```python
from build123d import *

# Parameters (mm, degrees)
BOSS_EXTRUDE1_DEPTH = 12
CUT_EXTRUDE1_DEPTH  = 20


with BuildPart() as part:
    # Sketch1 → Boss-Extrude1 (new body)
    with BuildSketch(Plane(origin=(0, 0, 0), x_dir=(1, 0, 0), z_dir=(0, 1, 0))):
        Polygon((0, 7.38), (-6.39126748, 3.69), (-6.39126748, -3.69), (0, -7.38), (6.39126748, -3.69), (6.39126748, 3.69), align=None)
    extrude(amount=BOSS_EXTRUDE1_DEPTH)

    # Sketch2 → Cut-Extrude1 (cut)
    with BuildSketch(Plane.XZ):
        Polygon((-2.165063509, -1.25), (2.165063509, -1.25), (0, 2.5), align=None)
    extrude(amount=-CUT_EXTRUDE1_DEPTH, mode=Mode.SUBTRACT)


solid = part.part
```
Verification items for the finished model (mm, model axes). A direction names the side the tool comes from. Coordinates: 2 decimals unless noted, no trailing zeros. Order: outer loops, then holes, each group sorted by start corner. A loop starts at its lowest first (then second) coordinate and runs counter-clockwise, first axis right, second up. Notation, with made-up numbers: (63, 12.5) - (79, 12.5) arc R21 cw to (79, 51.5) - close; hole circle Ø10 at (55, -30). An arc over 180 degrees is marked (long way). Return JSON: item names as keys, results as strings.
(1) Go/stop test with flat-tipped pins: pin 1 (6 mm diameter, centred on x = -1, y = 3, fed in from +Z); pin 2 (6 mm diameter, centred on x = -3.5, y = 9.5, fed in from -Z); pin 3 (5 mm diameter, centred on x = 3.5, z = -5.5, fed in from -Y). Record where each tip stops, or that it passes through.
Filled sheet:
{"pin 1": "stops at z = 7.38", "pin 2": "stops at z = -7.09", "pin 3": "stops at y = 0"}
(2) Mould release check, pull along X, two halves, no side actions. Record for faces 1 (the flat face through (-2, 0, 0)), 2 (the flat face through (3.24, 5.92, -5.51)), 3 (the flat face through (-1.07, 5.92, 0.65)): pulls with the +X half, pulls with the -X half, needs draft (parallel to the pull), parting line crosses it, or undercut.
Filled sheet:
{"face 1": "needs draft", "face 2": "pulls with the +X half", "face 3": "undercut"}
(3) Thickness scan on line 1 along Z through (x, y) = (-1, 1); line 2 along Z through (x, y) = (0.25, 4.5); line 3 along X through (y, z) = (2, 1.5). Record the ranges inside material, lowest first.
Filled sheet:
{"line 1": "z = -6.8 to -1.25, 0.77 to 6.8", "line 2": "z = -7.24 to -1.25, 2.07 to 7.24", "line 3": "x = -6.39 to -0.58, 0.58 to 6.39"}
(4) Section check D-D, the plane x = -3. Record the cut outline in (y, z), and give its area (3 significant figures).
Filled sheet:
{"outline": "(0, -5.65) - (12, -5.65) - (12, 5.65) - (0, 5.65) - close", "area": "136 mm^2"}
(5) Section check C-C, the plane z = 5. Record the cut outline in (x, y).
Filled sheet:
{"outline": "(-4.12, 0) - (4.12, 0) - (4.12, 12) - (-4.12, 12) - close"}
(6) Section check B-B, the plane x = -0.5. Record the cut outline in (y, z), and give its area (3 significant figures).
Filled sheet:
{"outline": "(0, -7.09) - (12, -7.09) - (12, -1.25) - (0, -1.25) - close; (0, 1.63) - (12, 1.63) - (12, 7.09) - (0, 7.09) - close", "area": "136 mm^2"}
(7) Access from +Z, -Z, +X, -X, +Y, -Y to the whole of each face (thin tool, end or side, straight path). Record for faces 4 (the flat face through (0, 6, -1.25)), 5 (the flat face through (6.391, 6, 0)).
Filled sheet:
{"face 4": "+Y, -Y", "face 5": "+Z, -Z, +X, +Y, -Y"}
(8) Section check A-A, the plane y = 9.75. Record the cut outline in (x, z).
Filled sheet:
{"outline": "(-6.39, -3.69) - (0, -7.38) - (6.39, -3.69) - (6.39, 3.69) - (0, 7.38) - (-6.39, 3.69) - close; hole (-2.17, -1.25) - (2.17, -1.25) - (0, 2.5) - close"}
